Geometry: final body of the model. Coordinates: model frame, mm. A direction names the side the tool comes from. Give positions to 0.01 mm unless a question says otherwise; leave off trailing zeros. Write each loop counter-clockwise with the first axis right and the second up, starting at its lowest first coordinate (ties: lowest second). Pieces come first, ordered by that corner, then holes.
Q1. Section D-D (x = -27.5). Return the cut outline in (y, z), plus the area to 3 significant figures.
Q2. Reachability of faces 4 (the flat face through (85, -29, 0)), 5 (the cylindrical face through (-48.747, 14.762, -4.974)), 6 (the flat face through (-87, 2, 0)) from +Z, -Z, +X, -X, +Y, -Y: full face, straight path, thin tool, end or side. Return the list, or none.
Q3. Pin query (flat end, axial travel): pin 1 Ø16 at (y, z) = (2.5, 4.5) entering from +X; pin 2 Ø1.2 at (y, z) = (-31.5, -3.5) entering from +X; pin 3 Ø2 at (x, y) = (110, -32.5) entering from -Z. Return the tip coordinate at first contact, or that it passes through.
Q4. Mould query, pull axis Y, two halves, no side actions, for faces 1 (the flat face through (100, -28, 0)), 2 (the flat face through (87, 2, 0)), 3 (the cylindrical face through (8.97, 2.54, -13.33)). Classes: +Y half, -Y half, draft (parallel to the pull), parting line (faces both ways), or undercut.
Q5. Section A-A (z = 0). State how many separate pieces and enclosed holes the cut face has, plus the area to 4 significant figures.
Q6. Section B-B (y = -21). Return the cut outline in (x, z).
Q7. Line query: line 1 (X direction, y = 29.25, z = 0); line 2 (Z direction, x = 73.5, y = -46.5); line 3 (X direction, y = 26.5, z = 7.5). Output: solid intervals per line, ascending.
Autodesk Inventor part; units mm, degrees
sketch "Sketch1" plane through (0, 0, 0) normal (0, 1, 0) x (-1, 0, 0)
  circle A0 centre (0, 0) radius 49
  dimension "d1" = 98
extrude "Extrusion1" add sketch "Sketch1" along normal blind 35
sketch "Sketch4" plane through (0, 35, 0) normal (0, 1, 0) x (1, 0, 0)
  circle A0 centre (0, 0) radius 47
  dimension "d8" = 94
extrude "Extrusion3" cut sketch "Sketch4" against normal blind 30
sketch "Sketch6" plane through (0, 35, 0) normal (0, 1, 0) x (1, 0, 0)
  circle A0 centre (0, 0) radius 49
  circle A1 centre (0, 0) radius 65
  dimension "d13" = 98
  dimension "d14" = 130
extrude "Extrusion4" add sketch "Sketch6" against normal blind 3
sketch "Sketch7" plane through (0, 5, 0) normal (0, 1, 0) x (1, 0, 0)
  line L0 (0, 68.6) -> (0, -68.6)
  line L1 (68.6, 0) -> (-68.6, 0)
  circle A0 centre (29.6304, 0) radius 14
  circle A1 centre (29.6304, 0) radius 15
  circle A2 centre (-20, -20) radius 14
  circle A3 centre (-20, -20) radius 15
  circle A4 centre (12, -27) radius 14
  circle A5 centre (12, -27) radius 15
  circle A6 centre (-20, 20) radius 14
  circle A7 centre (-20, 20) radius 15
  circle A8 centre (12, 27) radius 14
  circle A9 centre (12, 27) radius 15
  circle A10 centre (-7.7127, -37.6577) radius 2.5
  circle A11 centre (40.5942, 15) radius 2.5
  circle A12 centre (-7.7127, 38.4017) radius 2.5
  point P0 (0, 0)
  point P1 (0, -19.7889)
  point P2 (0, -34.2111)
  point P3 (0, 34.2111)
  point P4 (0, 19.7889)
  dimension "d92" = 28
  dimension "d93" = 30
  dimension "d94" = 28
  dimension "d95" = 30
  dimension "d96" = 28
  dimension "d97" = 30
  dimension "d98" = 28
  dimension "d99" = 30
  dimension "d100" = 28
  dimension "d101" = 30
  dimension "d102" = 20
  dimension "d103" = 20
  dimension "d104" = 20
  dimension "d105" = 20
  dimension "d106" = 12
  dimension "d107" = 27
  dimension "d108" = 12
  dimension "d109" = 27
  dimension "d110" = 5
  dimension "d111" = 5
  dimension "d112" = 5
extrude "Extrusion5" cut sketch "Sketch7" against normal through all contours A8 L0 | L0 A8 | A4 L0 | L0 A4 | A0 L1 | L1 A0 | A2 | A6 | A10 | A11 | A12
sketch "Sketch9" plane through (0, 35, 0) normal (0, 1, 0) x (1, 0, 0)
  circle A0 centre (0, 0) radius 65
  arc A1 (64.2262, -10) -> (64.2262, 10) centre (0, 0) ccw
  line L0 (64.2262, 10) -> (90, 10)
  line L1 (64.2262, -10) -> (90, -10)
  line L2 (90, -10) -> (90, 10)
  line L3 (121, 0) -> (-96, 0)
  point P0 (77.1131, 10)
  dimension "d41" = 10
  dimension "d42" = 20
  dimension "d43" = 90
extrude "Extrusion6" add sketch "Sketch9" against normal blind 3 contours L3 L2 L1 A0 | A0 L0 L2 L3
mirror "Mirror1" about plane through (0, 0, 0) normal (1, 0, 0) of "Extrusion6"
sketch "Sketch10" plane through (0, 32, 0) normal (0, -1, 0) x (1, 0, 0)
  line L0 (-90, 10) -> (-90, -10)
  line L1 (-90, 10) -> (-87, 10)
  line L2 (-87, 10) -> (-87, -10)
  line L3 (-87, -10) -> (-90, -10)
  line L4 (-90, -10) -> (-90, 10)
  point P0 (0, 0)
  dimension "d44" = 3
extrude "Extrusion7" add sketch "Sketch10" along normal blind 65
sketch "Sketch12" plane through (-90, 35, -10) normal (-1, 0, 0) x (0, 0, 1)
  circle A0 centre (10, -60) radius 6.5
  line L0 (20, -68) -> (0, -68)
  point P0 (10, -35)
  dimension "d49" = 13
  dimension "d50" = 8
extrude "Extrusion9" cut sketch "Sketch12" against normal blind 3
sketch "Sketch13" plane through (-87, 32, 10) normal (1, 0, 0) x (0, 0, -1)
  circle A0 centre (10, -57) radius 6.5
  arc A1 (5, -61.1533) -> (15, -61.1533) centre (10, -57) ccw
  line L0 (10, -78.6) -> (10, 16.6)
  line L1 (5, -61.1533) -> (0, -61.1533)
  line L2 (0, 0) -> (0, -65)
  line L3 (20, 0) -> (20, -65)
  line L4 (0, -65) -> (20, -65)
  line L5 (20, -65) -> (20, -61.1533)
  line L6 (15, -61.1533) -> (20, -61.1533)
  point P0 (10, -32)
  dimension "d53" = 5
  dimension "d54" = 5
extrude "Extrusion10" add sketch "Sketch13" along normal blind 15 and the other way blind 15 contours L6 L3 L4 L0 A0 | L0 L4 L2 L1 A0
sketch "Sketch18" plane through (0, 0, 0) normal (0, -1, 0) x (1, 0, 0)
  circle A0 centre (0, 0) radius 49
  circle A1 centre (-20, 20) radius 14
  circle A2 centre (-20, -20) radius 14
  line L0 (10.4184, -6.0653) -> (41.9411, -25.3366)
  line L1 (10.4184, -6.0653) -> (6.9184, -6.0653)
  line L2 (6.9184, -6.0653) -> (40.9681, -26.8814)
  arc A3 (40.8578, 27.0489) -> (39.6703, 28.7622) centre (0, 0) ccw
  arc A4 (40.9681, -26.8814) -> (41.9411, -25.3366) centre (0, 0) ccw
  line L3 (0, 0) -> (49, 0)
  line L4 (10.4184, 6.0653) -> (41.9411, 25.3366)
  line L5 (10.4184, 6.0653) -> (6.9184, 6.0653)
  line L6 (6.9184, 6.0653) -> (40.9681, 26.8814)
  arc A5 (41.9411, 25.3366) -> (40.9681, 26.8814) centre (0, 0) ccw
  dimension "d115" = 3.5
extrude "Extrusion15" add sketch "Sketch18" along normal blind 70 contours L4 L5 L6 A0 | A0 L2 L1 L0
sketch "Sketch19" plane through (0, 32, 0) normal (0, -1, 0) x (1, 0, 0)
  line L0 (90, -10) -> (64.2262, -10)
  line L1 (90, 10) -> (87, 10)
  line L2 (87, 10) -> (87, -10)
  line L3 (87, -10) -> (90, -10)
  line L4 (90, -10) -> (90, 10)
  point P0 (0, 0)
  dimension "d118" = 3
extrude "Extrusion16" add sketch "Sketch19" along normal blind 80
sketch "Sketch20" plane through (90, 35, 10) normal (1, 0, 0) x (0, 0, -1)
  line L0 (0, -3) -> (0, -64.1533)
  line L1 (20, 0) -> (20, -83)
  line L2 (0, -63) -> (20, -63)
  line L3 (20, -63) -> (20, -83)
  line L4 (20, -83) -> (0, -83)
  line L5 (0, -83) -> (0, -63)
  line L6 (1, -64) -> (19, -64)
  line L7 (19, -64) -> (19, -82)
  line L8 (19, -82) -> (1, -82)
  line L9 (1, -82) -> (1, -64)
  point P0 (10, -35)
  dimension "d121" = 20
  dimension "d122" = 18
  dimension "d123" = 18
  dimension "d124" = 19
  dimension "d125" = 1
extrude "Extrusion17" cut sketch "Sketch20" against normal blind 3 contours L6 L7 L8 L9
sketch "Sketch21" plane through (90, 35, 10) normal (1, 0, 0) x (0, 0, -1)
  line L0 (19, -64) -> (1, -64)
  line L1 (19, -82) -> (19, -64)
  line L2 (1, -64) -> (19, -64)
  line L3 (19, -64) -> (19, -82)
  line L4 (19, -82) -> (1, -82)
  line L5 (1, -82) -> (1, -64)
  line L6 (0, -3) -> (0, -83)
  line L7 (0, -83) -> (20, -83)
  line L8 (0, -63) -> (20, -63)
  line L9 (20, -63) -> (20, -83)
  line L10 (20, -83) -> (0, -83)
  line L11 (0, -83) -> (0, -63)
  point P0 (10, -35)
  dimension "d128" = 20
extrude "Extrusion18" add sketch "Sketch21" along normal blind 20 and the other way blind 30
sketch "Sketch22" plane through (110, 35, 10) normal (1, 0, 0) x (0, 0, -1)
  line L0 (0, -63) -> (20, -63)
  line L1 (20, -63) -> (20, -83)
  line L2 (0, -63) -> (20, -63)
  line L3 (20, -63) -> (20, -83)
  line L4 (20, -83) -> (0, -83)
  line L5 (0, -83) -> (0, -63)
  point P0 (10, -35)
extrude "Extrusion19" add sketch "Sketch22" along normal blind 1
sketch "Sketch23" plane through (111, 35, 10) normal (1, 0, 0) x (0, 0, -1)
  line L0 (2.5, -65.5) -> (17.5, -65.5)
  line L1 (17.5, -65.5) -> (17.5, -69.5)
  line L2 (17.5, -69.5) -> (2.5, -69.5)
  line L3 (2.5, -69.5) -> (2.5, -65.5)
  line L4 (10, -126) -> (10, 21)
  line L5 (0, -83) -> (20, -83)
  circle A0 centre (16, -79.5) radius 1
  line L6 (20, -83) -> (20, -63)
  circle A1 centre (4, -79.5) radius 1
  line L7 (0, -63) -> (0, -83)
  point P0 (10, -35)
  point P1 (17.5, -67.5)
  dimension "d135" = 15
  dimension "d136" = 7.5
  dimension "d137" = 4
  dimension "d138" = 17.5
  dimension "d139" = 10
  dimension "d140" = 2
  dimension "d141" = 4
  dimension "d142" = 2
  dimension "d143" = 10
  dimension "d144" = 4
extrude "Extrusion20" cut sketch "Sketch23" against normal blind 1
sketch "Sketch24" plane through (90, -28, 10) normal (0, 1, 0) x (1, 0, 0)
  line L0 (21, 20) -> (21, 0)
  line L1 (19, 17.5) -> (21, 17.5)
  line L2 (21, 17.5) -> (21, 2.5)
  line L3 (21, 2.5) -> (19, 2.5)
  line L4 (19, 2.5) -> (19, 17.5)
  line L5 (0, 0) -> (21, 0)
  point P0 (-90, 10)
  dimension "d147" = 15
  dimension "d148" = 2.5
  dimension "d149" = 2
extrude "Extrusion21" cut sketch "Sketch24" against normal blind 4
properties part number "VialHolder"
Computed:
1. outline: (0, -40.56) - (32, -40.56) - (32, -58.9) - (35, -58.9) - (35, -38.11) - (5, -38.11) - (5, -31.82) - (0, -31.82) - close; (0, -8.18) - (5, -8.18) - (5, 8.18) - (0, 8.18) - close; (0, 31.82) - (5, 31.82) - (5, 38.11) - (35, 38.11) - (35, 58.9) - (32, 58.9) - (32, 40.56) - (0, 40.56) - close
1. area: 426 mm2
2. face 4: none
2. face 5: -Y
2. face 6: +Z, -Z
3. pin 1: stops at x = 90
3. pin 2: stops at x = -72
3. pin 3: stops at z = -10
4. face 1: +Y half
4. face 2: undercut
4. face 3: draft
5. separate pieces: 4
5. enclosed holes: 0
5. area: 1,205 mm2
6. outline: (-90, -10) - (-87, -10) - (-87, -5.12) - (-90, -5.12) - close; (-90, 5.12) - (-87, 5.12) - (-87, 10) - (-90, 10) - close; (6.92, -6.07) - (40.97, -26.88) arc R49 ccw to (41.94, -25.34) - (10.42, -6.07) - close; (6.92, 6.07) - (10.42, 6.07) - (41.94, 25.34) arc R49 ccw to (40.97, 26.88) - close; (87, -10) - (90, -10) - (90, 10) - (87, 10) - close
7. line 1: x = -90 to -87, -49 to -47, 47 to 49, 87 to 90
7. line 2: z = -10 to -9, 9 to 10
7. line 3: x = -90 to -87, -48.42 to -46.4, 46.4 to 48.42, 87 to 90
